Here's how the part is built. I have some questions about the finished solid (model axes, mm). Face numbers are marked on the shaded views. A direction names the side the tool comes from. Coordinates: 2 decimals unless noted, no trailing zeros. Loops run counter-clockwise (first coordinate to the right, second up) from the corner with the lowest first, then second, coordinate; pieces in that order, holes last.
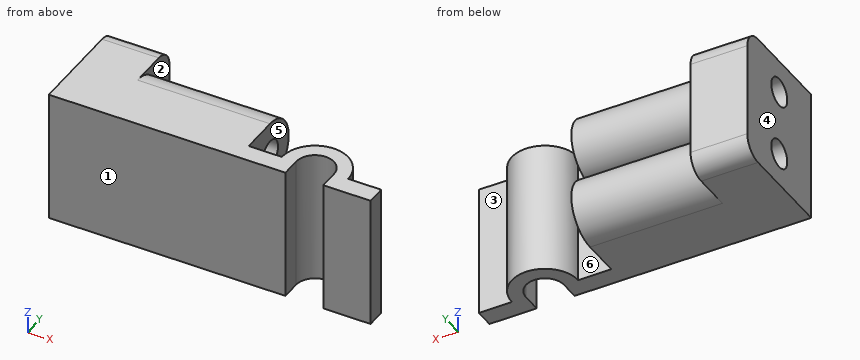
```python
from build123d import *

# Parameters (mm, degrees)
BOSS_EXTRUDE1_DEPTH = 70
FILLET1_R           = 10
FILLET2_R           = 10
BOSS_EXTRUDE2_DEPTH = 70
SKETCH3_R           = 7.5
CUT_EXTRUDE1_DEPTH  = 185


with BuildPart() as part:
    # Sketch1 → Boss-Extrude1 (new body)
    with BuildSketch(Plane.XY):
        with BuildLine():
            Line((67.5, -20), (85, -20))
            Line((85, -20), (85, -30))
            Line((85, -30), (60, -30))
            Line((60, -30), (60, -20))
            ThreePointArc((60, -20), (50, -10), (40, -20))
            Line((40, -20), (40, -30))
            Line((40, -30), (-85, -30))
            Line((-85, -30), (-85, 30))
            Line((-85, 30), (-55, 30))
            Line((-55, 30), (-55, 0))
            Line((-55, 0), (15, 0))
            Line((15, 0), (15, -20))
            Line((15, -20), (32.5, -20))
            ThreePointArc((32.5, -20), (50, -2.5), (67.5, -20))
        make_face()
    extrude(amount=-BOSS_EXTRUDE1_DEPTH)

    # Fillet1
    fillet1_edges = [part.edges().sort_by_distance(p)[0] for p in [
        (-70, 30, 0),
    ]]
    fillet(fillet1_edges, radius=FILLET1_R)

    # Fillet2
    fillet2_edges = [part.edges().sort_by_distance(p)[0] for p in [
        (-70, 30, -70),
    ]]
    fillet(fillet2_edges, radius=FILLET2_R)

    # Sketch2 → Boss-Extrude2 (add)
    with BuildSketch(Plane(origin=(15, 0, 0), x_dir=(0, 0, -1), z_dir=(1, 0, 0))):
        with BuildLine():
            ThreePointArc((35, 0), (17.5, 17.5), (0, 0))
            Line((0, 0), (35, 0))
        make_face()
        with BuildLine():
            ThreePointArc((70, 0), (52.5, 17.5), (35, 0))
            Line((35, 0), (70, 0))
        make_face()
    extrude(amount=-BOSS_EXTRUDE2_DEPTH)

    # Sketch3 → Cut-Extrude1 (cut)
    with BuildSketch(Plane(origin=(15, 0, 0), x_dir=(0, 0, -1), z_dir=(1, 0, 0))):
        with Locations(Location((17.5, 0, 0), (0, 0, 90))):
            Circle(SKETCH3_R)
        with Locations(Location((52.5, 0, 0), (0, 0, 90))):
            Circle(SKETCH3_R)
    extrude(amount=-CUT_EXTRUDE1_DEPTH, mode=Mode.SUBTRACT)


solid = part.part
```
1. I want a section at A-A (x = -5.5). Please give me the cut outline in (y, z), then the cut area to 3 significant figures.
2. I want a section at C-C (y = -18). Please give me the cut outline in (x, z).
3. I want a section at B-B (z = -52.5). Please give me the cut outline in (x, y), then the cut area to 3 significant figures.
4. I want a section at D-D (y = 12.5). Please give me the cut outline in (x, z).
5. We'd pull the mould along X, two halves only. Please class the marked faces 3, 4, 5 and 6: +X half, -X half, draft (parallel to the pull), parting line (faces both ways), or undercut.
6. On a 3-axis mill with a long thin cutter (end or side, diameter ignored), from which of +Z, -Z, +X, -X, +Y, -Y can I reach the whole of each face in a straight line? I mean the marked faces 1 and 2. Say none if no direction works.
7. I need wall thicknesses on line 1 along X through (y, z) = (-19.5, -17.5); line 2 along X through (y, z) = (-25, -21); line 3 along X through (y, z) = (-16, -16). Which ranges of each line are inside material? Lowest first, please.
8. For pin 1 (5 mm diameter, centred on x = 73, z = -40, fed in from +Y); pin 2 (19.5 mm diameter, centred on y = 0, z = -17.5, fed in from +X); pin 3 (8 mm diameter, centred on x = 46.5, z = -62.5, fed in from +Y), each with a flat end and sliding along its axis, tell me the tip position at first contact or that it passes through.
Response values:
1. outline: (-30, -70) - (0, -70) arc R17.5 ccw to (0, -35) arc R17.5 ccw to (0, 0) - (-30, 0) - close; hole circle Ø15 at (0, -52.5); hole circle Ø15 at (0, -17.5)
1. area: 2,710 mm2
2. outline: (-85, -70) - (15, -70) - (15, 0) - (-85, 0) - close; (32.61, -70) - (40.2, -70) - (40.2, 0) - (32.61, 0) - close; (59.8, -70) - (67.39, -70) - (67.39, 0) - (59.8, 0) - close
3. outline: (-85, -30) - (40, -30) - (40, -20) arc R10 cw to (60, -20) - (60, -30) - (85, -30) - (85, -20) - (67.5, -20) arc R17.5 ccw to (32.5, -20) - (15, -20) - (15, -7.5) - (-85, -7.5) - close; (-85, 7.5) - (15, 7.5) - (15, 17.5) - (-55, 17.5) - (-55, 30) - (-85, 30) - close
3. area: 4,450 mm2
4. outline: (-85, -70) - (-55, -70) - (-55, -64.75) - (15, -64.75) - (15, -40.25) - (-55, -40.25) - (-55, -29.75) - (15, -29.75) - (15, -5.25) - (-55, -5.25) - (-55, 0) - (-85, 0) - close
5. face 3: draft
5. face 4: -X half
5. face 5: undercut
5. face 6: undercut
6. face 1: +Z, -Z, +X, -X, -Y
6. face 2: +X, +Y
7. line 1: x = -85 to 15, 32.51 to 40.01, 59.99 to 67.49
7. line 2: x = -85 to 40, 60 to 85
7. line 3: x = -85 to 15, 32.96 to 40.83, 59.17 to 67.04
8. pin 1: stops at y = -20
8. pin 2: stops at x = 64.18
8. pin 3: stops at y = -2.5
